from build123d import *

# Parameters (mm, degrees)
MODEL_W             = 90
MODEL_H             = 122
BOSS_EXTRUDE1_DEPTH = 15
MODEL_3_W           = 89
MODEL_3_H           = 121
BOSS_EXTRUDE2_DEPTH = 1.6
BOSS_EXTRUDE3_DEPTH = 10
MODEL_5_W           = 7.6
MODEL_5_H           = 10
BOSS_EXTRUDE4_DEPTH = 10
MODEL_6_W           = 7.6
MODEL_6_H           = 30
BOSS_EXTRUDE5_DEPTH = 10
MODEL_7_R           = 2.5
CUT_EXTRUDE1_DEPTH  = 10
SKETCH4_R           = 4.955800122
CUT_EXTRUDE2_DEPTH  = 2


with BuildPart() as part:
    # Model → Boss-Extrude1 (new body)
    with BuildSketch(Plane.XY):
        Rectangle(MODEL_W, MODEL_H)
    extrude(amount=-BOSS_EXTRUDE1_DEPTH)

    # Model_3 → Boss-Extrude2 (add)
    with BuildSketch(Plane.XY):
        Rectangle(MODEL_3_W, MODEL_3_H)
    extrude(amount=BOSS_EXTRUDE2_DEPTH)

    # Model_4 → Boss-Extrude3 (add)
    with BuildSketch(Plane.XY):
        Polygon((-35, 45.958548116), (-31.5, 47.979274058), (-31.5, 52.020725942), (-35, 54.041451884), (-38.5, 52.020725942), (-38.5, 47.979274058), align=None)
        Polygon((35, 45.958548116), (38.5, 47.979274058), (38.5, 52.020725942), (35, 54.041451884), (31.5, 52.020725942), (31.5, 47.979274058), align=None)
        Polygon((35, -45.958548116), (31.5, -47.979274058), (31.5, -52.020725942), (35, -54.041451884), (38.5, -52.020725942), (38.5, -47.979274058), align=None)
        Polygon((-35, -45.958548116), (-38.5, -47.979274058), (-38.5, -52.020725942), (-35, -54.041451884), (-31.5, -52.020725942), (-31.5, -47.979274058), align=None)
    extrude(amount=BOSS_EXTRUDE3_DEPTH)

    # Model_5 → Boss-Extrude4 (add)
    with BuildSketch(Plane.XY):
        with Locations((-39.8, 17.5)):
            Rectangle(MODEL_5_W, MODEL_5_H)
        with Locations((39.8, 17.5)):
            Rectangle(MODEL_5_W, MODEL_5_H)
    extrude(amount=BOSS_EXTRUDE4_DEPTH)

    # Model_6 → Boss-Extrude5 (add)
    with BuildSketch(Plane.XY):
        with Locations((-39.8, -7.5)):
            Rectangle(MODEL_6_W, MODEL_6_H)
        with Locations((39.8, -7.5)):
            Rectangle(MODEL_6_W, MODEL_6_H)
    extrude(amount=BOSS_EXTRUDE5_DEPTH)

    # Model_7 → Cut-Extrude1 (cut)
    with BuildSketch(Plane.XY):
        with Locations((-35, 50)):
            Circle(MODEL_7_R)
        with Locations((35, 50)):
            Circle(MODEL_7_R)
        with Locations((-35, -50)):
            Circle(MODEL_7_R)
        with Locations((35, -50)):
            Circle(MODEL_7_R)
    extrude(amount=CUT_EXTRUDE1_DEPTH, mode=Mode.SUBTRACT)

    # Sketch4 → Cut-Extrude2 (cut)
    with BuildSketch(Plane(origin=(0, 0, -15), x_dir=(-1, 0, 0), z_dir=(0, 0, -1))):
        with Locations((31.0232, -47.0464)):
            Circle(SKETCH4_R)
        Polygon((25.369, 0.0335), (19.9902, 4.7816), (-17.1378, 4.8101), (-23.6203, 0.0312), (-19.0147, -4.0613), (19.1392, -4.0613), align=None)
        Polygon((-37.1536, -42.7978), (-36.13, -44.9525), (-29.1472, -39.6744), (-22.2668, -5.0611), (-26.7704, -1.1876), (-30.8986, -4.3118), (-38.029, -40.7988), align=None)
        Polygon((-19.7654, 5.9353), (-12.654031371, 40.081219045), (-17.3886, 48.2956), (-18.8893, 46.9206), (-20.0154, 45.2958), (-20.8906, 43.5466), (-21.3914, 41.5476), (-29.0226, 3.56045), (-25.7696, 1.5615), align=None)
        Polygon((-10.7582, 40.4232), (26.2696, 40.4232), (33.6508, 47.2956), (31.0232, 48.9196), (28.271, 50.0448), (-11.259, 50.0448), (-13.5104, 49.9194), (-15.8871, 49.1702), align=None)
        Polygon((22.3922, 6.4348), (27.3956, 2.061), (31.5238, 4.8101), (38.013524934, 40.463880597), (37.2782, 42.4222), (36.152, 44.1714), (34.9014, 45.9206), (29.1472, 40.4232), align=None)
        Polygon((20.14, -6.9356), (13.3477, -39.4168), (18.3604, -47.3956), (21.016, -44.298), (29.647, -3.5617), (27.771, -1.937), align=None)
        Polygon((12.7596, -49.5456), (-30.2732, -49.5456), (-34.276, -47.0464), (-26.2704, -40.8369), (11.8843, -40.7988), (16.652, -48.4566), align=None)
    extrude(amount=-CUT_EXTRUDE2_DEPTH, mode=Mode.SUBTRACT)


solid = part.part
Design review of the part built by this model. Coordinates are the model's own, in mm. A direction names the side the tool comes from. Coordinates: 2 decimals unless noted, no trailing zeros. Order: outer loops, then holes, each group sorted by start corner. A loop starts at its lowest first (then second) coordinate and runs counter-clockwise, first axis right, second up. Notation, with made-up numbers: (27, -30.5) - (81, -30.5) arc R17 cw to (81, -0.5) - close; hole circle Ø2 at (79, 74.5). An arc over 180 degrees is marked (long way). Put each result on its own line as item: value.
1) Wall thickness on L1, parallel to Y at x = -35, z = 2.5; L2, parallel to Y at x = -35.5, z = 7.5; L3, parallel to X at y = -48, z = 8.25: over which ranges is each line inside the solid? List them lowest first. Write a range as from..to.
Response values:
L1: y = -54.04..-52.5, -47.5..-45.96, 45.96..47.5, 52.5..54.04
L2: y = -53.75..-52.45, -47.55..-46.25, 46.25..47.55, 52.45..53.75
L3: x = -38.5..-36.5, -33.5..-31.5, 31.5..33.5, 36.5..38.5
2) Tool access review of faces 1 (the face through (25.755, -22.61, -14.014)), 2 (the face through (-36, 17, 6)), 3 (the face through (-31.5, 50, 6)), 4 (the face through (43.6, 17, 6)): name each direction out of +Z, -Z, +X, -X, +Y, -Y from which nothing blocks a thin tool from reaching the whole face with its end or side.
Response values:
face 1: -Z
face 2: +Z
face 3: +Z, +Y, -Y
face 4: +Z, +X, +Y, -Y
3) Take a section at A-A, the plane y = 24.5. Give the boundary of the cut face in (x, z).
Response values:
outline: (-45, -15) - (-35.11, -15) - (-35.11, -13) - (-25.98, -13) - (-25.98, -15) - (15.9, -15) - (15.9, -13) - (24.82, -13) - (24.82, -15) - (45, -15) - (45, 0) - (44.5, 0) - (44.5, 1.6) - (-44.5, 1.6) - (-44.5, 0) - (-45, 0) - close
4) Insertion check: P1, Ø6, axis at x = 39, z = 7, coming from the -Y side; P2, Ø2, axis at y = 50, z = 5, coming from the -X side; P3, Ø4, axis at x = -39.5, z = 4, coming from the -Y side; P4, Ø5, axis at x = -4.5, z = 5.5, coming from the -Y side. Each pin has a flat end and moves straight along its axis. Give the tip position at first contact, or say it passes through.
Response values:
P1: stops at y = -53.46
P2: stops at x = -38.5
P3: stops at y = -52.6
P4: passes through
5) Take a section at D-D, the plane y = -36. Give the boundary of the cut face in (x, z).
Response values:
outline: (-45, -15) - (-22.77, -15) - (-22.77, -13) - (-14.06, -13) - (-14.06, -15) - (28.42, -15) - (28.42, -13) - (37.09, -13) - (37.09, -15) - (45, -15) - (45, 0) - (44.5, 0) - (44.5, 1.6) - (-44.5, 1.6) - (-44.5, 0) - (-45, 0) - close
6) Take a section at B-B, the plane x = 1.5. Give the boundary of the cut face in (y, z), and give its area (3 significant figures).
Response values:
outline: (-61, -15) - (-49.55, -15) - (-49.55, -13) - (-40.81, -13) - (-40.81, -15) - (-4.06, -15) - (-4.06, -13) - (4.8, -13) - (4.8, -15) - (40.42, -15) - (40.42, -13) - (50.04, -13) - (50.04, -15) - (61, -15) - (61, 0) - (60.5, 0) - (60.5, 1.6) - (-60.5, 1.6) - (-60.5, 0) - (-61, 0) - close
area: 1,970 mm²
7) Take a section at C-C, the plane y = -15. Give the boundary of the cut face in (x, z), and give its area (3 significant figures).
Response values:
outline: (-45, -15) - (-27.22, -15) - (-27.22, -13) - (-18.45, -13) - (-18.45, -15) - (24.24, -15) - (24.24, -13) - (32.99, -13) - (32.99, -15) - (45, -15) - (45, 0) - (44.5, 0) - (44.5, 1.6) - (43.6, 1.6) - (43.6, 10) - (36, 10) - (36, 1.6) - (-36, 1.6) - (-36, 10) - (-43.6, 10) - (-43.6, 1.6) - (-44.5, 1.6) - (-44.5, 0) - (-45, 0) - close
area: 1,590 mm²
8) The part is to be moulded in two halves that separate along Y. For faces 5 (the face through (-43.6, 17, 6)), 6 (the face through (-22.21, -2.043, -14.014)), 7 (the face through (-25.27, -24.22, -14.01)), 8 (the face through (-33.274, -53.045, 5.741)), say which applies: released by +Y, released by -Y, zero draft, split by the parting line, or undercut.
Response values:
face 5: zero draft
face 6: undercut
face 7: undercut
face 8: released by -Y
